```python
from build123d import *

# Parameters (mm, degrees)
SKETCH_1_W      = 20
SKETCH_1_H      = 120
EXTRUDE_1_DEPTH = 20
EXTRUDE_2_DEPTH = 20


with BuildPart() as part:
    # 草图1 → 凸台-拉伸1 (new body)
    with BuildSketch(Plane(origin=(0, 0, 0), x_dir=(1, 0, 0), z_dir=(0, 1, 0))):
        Rectangle(SKETCH_1_W, SKETCH_1_H)
    extrude(amount=EXTRUDE_1_DEPTH)

    # 草图2 → 凸台-拉伸2 (add)
    with BuildSketch(Plane(origin=(10, 0, 0), x_dir=(0, 0, -1), z_dir=(1, 0, 0))):
        Polygon((0, 20), (40, 20), (40, 70), (-40, 70), (-40, 20), align=None)
    extrude(amount=-EXTRUDE_2_DEPTH)


solid = part.part
```
Can you work these out from the model? Positions are in its coordinate system, mm. A direction names the side the tool comes from. Coordinates: 2 decimals unless noted, no trailing zeros. Order: outer loops, then holes, each group sorted by start corner. A loop starts at its lowest first (then second) coordinate and runs counter-clockwise, first axis right, second up. Notation, with made-up numbers: (48, 11) - (91, 11) arc R19 cw to (91, 35) - close; hole circle Ø5 at (82, 68). An arc over 180 degrees is marked (long way). Answer in a Markdown table with one row per item.
1. Suppose I cut it at B-B (y = 62). Please give me the cut outline in (x, z), and give its area (3 significant figures).
Reply:
| item | result |
|---|---|
| outline | (-10, -40) - (10, -40) - (10, 40) - (-10, 40) - close |
| area | 1,600 mm^2 |
2. Suppose I cut it at A-A (x = -1.25). Please give me the cut outline in (y, z), and give its area (3 significant figures).
Reply:
| item | result |
|---|---|
| outline | (0, -60) - (20, -60) - (20, -40) - (70, -40) - (70, 40) - (20, 40) - (20, 60) - (0, 60) - close |
| area | 6,400 mm^2 |
3. For pin 1 (1 mm diameter, centred on x = -6, z = -45, fed in from +Y); pin 2 (10 mm diameter, centred on x = -0.5, y = 42.5, fed in from -Z), each with a flat end and sliding along its axis, tell me the tip position at first contact or that it passes through.
Reply:
| item | result |
|---|---|
| pin 1 | stops at y = 20 |
| pin 2 | stops at z = -40 |
4. If I drill on line 1 along Z through (x, y) = (7.75, 40); line 2 along Y through (x, z) = (-9, 46), over which ranges is the centre line in solid material (lowest first)?
Reply:
| item | result |
|---|---|
| line 1 | z = -40 to 40 |
| line 2 | y = 0 to 20 |
5. For faces 1 (the flat face through (10, 35, 1)), 2 (the flat face through (0, 20, 50)), 3 (the flat face through (0, 20, -50)), which set-ups out of +Z, -Z, +X, -X, +Y, -Y let a thin tool reach every point of the face, with its end or its side?
Reply:
| item | result |
|---|---|
| face 1 | +Z, -Z, +X, +Y, -Y |
| face 2 | +Z, +X, -X, +Y |
| face 3 | -Z, +X, -X, +Y |
6. Suppose I cut it at C-C (z = 52.5). Please give me the cut outline in (x, y).
Reply:
| item | result |
|---|---|
| outline | (-10, 0) - (10, 0) - (10, 20) - (-10, 20) - close |
